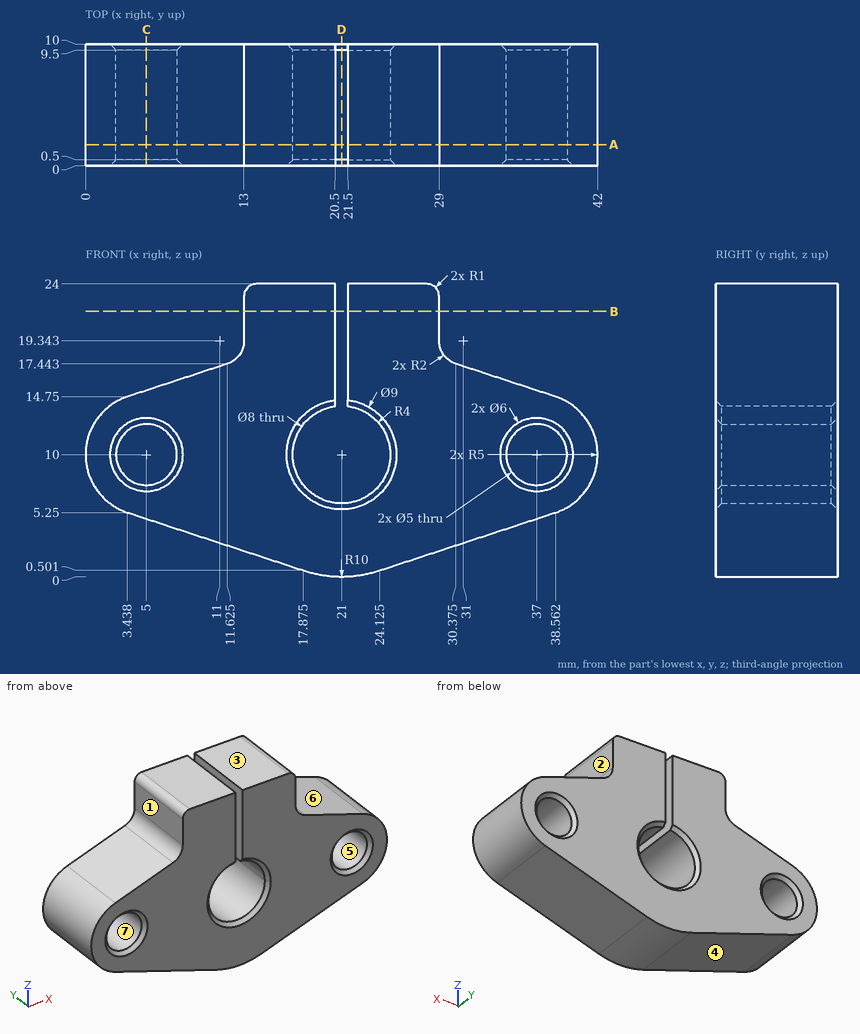
Can you work these out from the drawing? Everything is in mm from the part's minimum corner. A direction names the side the tool comes from. Coordinates: 2 decimals unless noted, no trailing zeros. Order: outer loops, then holes, each group sorted by start corner. A loop starts at its lowest first (then second) coordinate and runs counter-clockwise, first axis right, second up. Notation, with made-up numbers: (-12, -17.75) -> (33, -17.75) arc R22 ccw to (33, 9.25) -> close; hole circle Ø3 at (2, 31.25). An arc over 180 degrees is marked (long way). Use one line per item in the form item = value.
Q1. Which directions (+Z, -Z, +X, -X, +Y, -Y) give clear straight access to the entire face, cutting with the end or side of a thin tool? Please do the marked faces 1, 2 and 3.
From the geometry:
face_1 = +Z, -X, +Y, -Y
face_2 = +Z, +X, +Y, -Y
face_3 = +Z, +X, -X, +Y, -Y
Q2. We'd pull the mould along X, two halves only. Please class the marked faces 4, 5, 6 and 7: released by +X, released by -X, zero draft, split by the parting line, or undercut.
From the geometry:
face_4 = released by -X
face_5 = undercut
face_6 = released by +X
face_7 = undercut
Q3. Imagine slicing it at A-A, the plane y = 1.75. Give the number of separate pieces and of enclosed holes in the cut face, then the cut area to 3 significant figures.
From the geometry:
separate_pieces = 1
enclosed_holes = 2
area = 561 mm²
Q4. Imagine slicing it at D-D, the plane x = 21. List the corners of the cut face in (y, z) for me.
From the geometry:
outline = (0, 0) -> (10, 0) -> (10, 5.5) -> (9.5, 6) -> (0.5, 6) -> (0, 5.5) -> close
Q5. Imagine slicing it at C-C, the plane x = 5. List the corners of the cut face in (y, z) for me.
From the geometry:
outline = (0, 4.74) -> (10, 4.74) -> (10, 7) -> (9.5, 7.5) -> (0.5, 7.5) -> (0, 7) -> close; (0, 13) -> (0.5, 12.5) -> (9.5, 12.5) -> (10, 13) -> (10, 15.26) -> (0, 15.26) -> close
Q6. Imagine slicing it at B-B, the plane z = 21.75. List the corners of the cut face in (x, y) for me, then the cut area to 3 significant figures.
From the geometry:
outline = (13, 0) -> (20.5, 0) -> (20.5, 10) -> (13, 10) -> close; (21.5, 0) -> (29, 0) -> (29, 10) -> (21.5, 10) -> close
area = 150 mm²
Q7. Will these pins go through, and if not, where does the flat tip stop? P1, Ø1.1, axis at y = 3, z = 21, coming from the -X side; P2, Ø5, axis at y = 1.5, z = 4, coming from the -X side; P3, Ø1, axis at x = 30.5, y = 1, coming from the -Z side; P4, Ø2, axis at x = 23.5, z = 9.5, coming from the +Y side.
From the geometry:
P1 = 13
P2 = 1.43
P3 = 2.43
P4 = through
Q8. I need wall thicknesses on L1, parallel to X at y = 2.25, z = 10.25; L2, parallel to X at y = 8.5, z = 21; L3, parallel to Z at x = 5, y = 3 (1 decimal). Which ranges of each line are inside material? Lowest first, please.
From the geometry:
L1 = 0.01 to 2.51, 7.49 to 17.01, 24.99 to 34.51, 39.49 to 41.99
L2 = 13 to 20.5, 21.5 to 29
L3 = 4.7 to 7.5, 12.5 to 15.3
